The model under review builds one solid part; all positions refer to its coordinate system, in mm. Face numbers are marked on the shaded views. Give positions to 0.01 mm unless a question says otherwise; leave off trailing zeros. Order: outer loops, then holes, each group sorted by start corner. A loop starts at its lowest first (then second) coordinate and runs counter-clockwise, first axis right, second up.
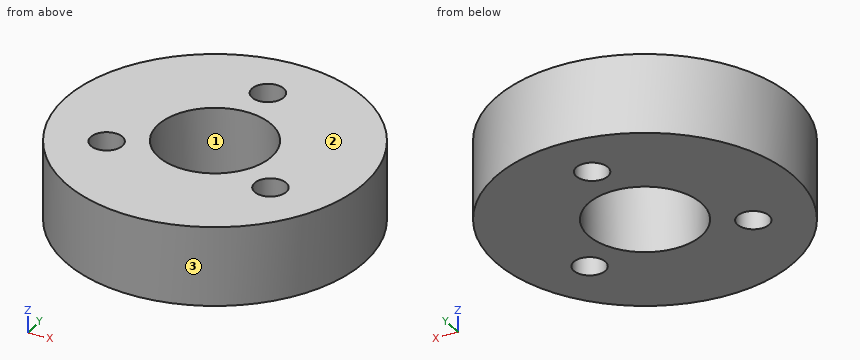
Autodesk Inventor part; units mm, degrees
ref_plane "Work Plane1" through (-191.7635, -303.2503, 17.5) normal (0, 0, -1) x (-0.1566, 0.9877, 0)
ref_plane "YZ Plane" through (0, 0, 0) normal (1, 0, 0) x (0, 1, 0)
ref_plane "XZ Plane" through (0, 0, 0) normal (0, 1, 0) x (-1, 0, 0)
sketch "Sketch1" plane through (0, 0, 0) normal (0, 0, 1) x (1, 0, 0)
  circle A0 centre (0, 20.7846) radius 3.5
  circle A1 centre (-18, -10.3923) radius 3.5
  circle A2 centre (18, -10.3923) radius 3.5
  circle A3 centre (0, 0) radius 6.75 construction
  circle A4 centre (0, 0) radius 12.5
  circle A5 centre (0, 0) radius 33
  point P0 (0, 0)
  dimension "d0" = 25
ref_plane "Work Plane1" through (-191.7635, -303.2503, 17.5) normal (0, 0, -1) x (-0.1566, 0.9877, 0)
extrude "Extrusion1" add sketch "Sketch1" along normal up to surface (17.5 mm away)
properties part number "LegMotorSpacer"
1. To check wall thickness, follow line 1 (Y direction, x = 0, z = 6); line 2 (X direction, y = -8, z = 12.5); line 3 (Y direction, x = 0.5, z = 7.5). State the ranges of each line that lie inside material, in increasing order.
2. Take a section at B-B (y = 0). Write out the cut boundary in (x, z), and give its area (4 significant figures).
3. Insertion check: pin 1 (4 mm diameter, centred on x = 10.5, z = 6.5, fed in from +Y); pin 2 (10 mm diameter, centred on x = 17.5, z = 9, fed in from -Y); pin 3 (6 mm diameter, centred on x = -23.5, z = 6.5, fed in from -Y). Each pin has a flat end and moves straight along its axis. Give the tip position at first contact, or say it passes through.
4. Take a section at C-C (x = -18). Write out the cut boundary in (y, z), and give its area (3 significant figures).
5. Take a section at D-D (z = 14). Write out the cut boundary in (x, y).
6. Take a section at A-A (x = 0). Write out the cut boundary in (y, z).
7. Draft analysis for pull direction Y (two halves, no side actions). For the marked faces 1, 2 and 3, state which applies: pulls with the +Y half, pulls with the -Y half, needs draft (parallel to the pull), parting line crosses it, or undercut.
Answer:
1. line 1: y = -33 to -12.5, 12.5 to 17.28, 24.28 to 33
1. line 2: x = -32.02 to -20.55, -15.45 to -9.6, 9.6 to 15.45, 20.55 to 32.02
1. line 3: y = -33 to -12.49, 12.49 to 17.32, 24.25 to 33
2. outline: (-33, 0) - (-12.5, 0) - (-12.5, 17.5) - (-33, 17.5) - close; (12.5, 0) - (33, 0) - (33, 17.5) - (12.5, 17.5) - close
2. area: 717.5 mm2
3. pin 1: stops at y = 31.89
3. pin 2: stops at y = -30.54
3. pin 3: stops at y = -25.86
4. outline: (-27.66, 0) - (-13.89, 0) - (-13.89, 17.5) - (-27.66, 17.5) - close; (-6.89, 0) - (27.66, 0) - (27.66, 17.5) - (-6.89, 17.5) - close
4. area: 846 mm2
5. outline: circle Ø66 at (0, 0); hole circle Ø7 at (-18, -10.39); hole circle Ø25 at (0, 0); hole circle Ø7 at (0, 20.78); hole circle Ø7 at (18, -10.39)
6. outline: (-33, 0) - (-12.5, 0) - (-12.5, 17.5) - (-33, 17.5) - close; (12.5, 0) - (17.28, 0) - (17.28, 17.5) - (12.5, 17.5) - close; (24.28, 0) - (33, 0) - (33, 17.5) - (24.28, 17.5) - close
7. face 1: undercut
7. face 2: needs draft
7. face 3: parting line crosses it
